Here's how the part is built. I have some questions about the finished solid (model axes, mm). Face numbers are marked on the shaded views. Give positions to 0.01 mm unless a question says otherwise; leave off trailing zeros. Loops run counter-clockwise (first coordinate to the right, second up) from the corner with the lowest first, then second, coordinate; pieces in that order, holes last. Notation, with made-up numbers: (4.25, 64) - (52.25, 64) arc R21 ccw to (52.25, 68) - close; hole circle Ø11 at (20, 48.5). An arc over 180 degrees is marked (long way). Use a Markdown table: item, result.
from build123d import *

# Parameters (mm, degrees)
ESQUISSE1_R             = 6
EXTRUSION1_DEPTH        = 30.5
CHANFREIN1_SIZE         = 1
CHANFREIN1_SIZE2        = 3.732050808
ESQUISSE2_R             = 2
ENL_V_MAT_EXTRU_1_DEPTH = 1


with BuildPart() as part:
    # Esquisse1 → Extrusion1 (new body)
    with BuildSketch(Plane(origin=(0, 0, 0), x_dir=(1, 0, 0), z_dir=(0, 1, 0))):
        Circle(ESQUISSE1_R)
    extrude(amount=EXTRUSION1_DEPTH)

    # Chanfrein1
    chanfrein1_edges = [part.edges().sort_by_distance(p)[0] for p in [
        (-6, 30.5, 0),
    ]]
    chanfrein1_side = [part.faces().sort_by_distance(p)[0] for p in [
        (-6, 15.25, 0),
    ]]
    chamfer(chanfrein1_edges, length=CHANFREIN1_SIZE, length2=CHANFREIN1_SIZE2, reference=chanfrein1_side[0])

    # Esquisse2 → Enlèv. mat.-Extru.1 (cut)
    with BuildSketch(Plane(origin=(0, 30.5, 0), x_dir=(1, 0, 0), z_dir=(0, 1, 0))):
        Circle(ESQUISSE2_R)
    extrude(amount=-ENL_V_MAT_EXTRU_1_DEPTH, mode=Mode.SUBTRACT)


solid = part.part
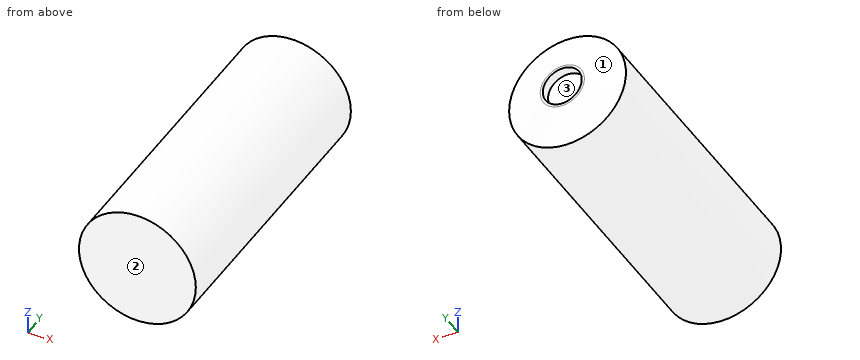
(1) We'd pull the mould along X, two halves only. Please class the marked faces 1, 2 and 3: pulls with the +X half, pulls with the -X half, needs draft (parallel to the pull), parting line crosses it, or undercut.
A:
| item | result |
|---|---|
| face 1 | parting line crosses it |
| face 2 | needs draft |
| face 3 | undercut |
(2) Suppose I cut it at A-A on x = 0. Write out the boundary of the cut face in (y, z), plus the area to 3 significant figures.
A:
| item | result |
|---|---|
| outline | (0, -6) - (29.5, -6) - (30.5, -2.27) - (30.5, -2) - (29.5, -2) - (29.5, 2) - (30.5, 2) - (30.5, 2.27) - (29.5, 6) - (0, 6) - close |
| area | 358 mm2 |
(3) Suppose I cut it at B-B on z = 0. Write out the boundary of the cut face in (x, y), plus the area to 3 significant figures.
A:
| item | result |
|---|---|
| outline | (-6, 0) - (6, 0) - (6, 29.5) - (2.27, 30.5) - (2, 30.5) - (2, 29.5) - (-2, 29.5) - (-2, 30.5) - (-2.27, 30.5) - (-6, 29.5) - close |
| area | 358 mm2 |
(4) If I drill on line 1 (Y direction, x = -0.25, z = -0.5); line 2 (Y direction, x = -5.5, z = 1.75); line 3 (Z direction, x = 3.75, y = 26), over which ranges is the centre line in solid material (lowest first)?
A:
| item | result |
|---|---|
| line 1 | 0 to 29.5 |
| line 2 | 0 to 29.56 |
| line 3 | -4.68 to 4.68 |
(5) Suppose I cut it at C-C on y = 4. Write out the boundary of the cut face in (x, z).
A:
| item | result |
|---|---|
| outline | circle Ø12 at (0, 0) |
(6) Will this pin go through, and if not, where does the flat tip stop? pin 1 (1.5 mm diameter, centred on x = 1, y = 20, fed in from -Z).
A:
| item | result |
|---|---|
| pin 1 | z = -5.99 |
